Verification items for the finished model (mm, model axes). A direction names the side the tool comes from. Give positions to 0.01 mm unless a question says otherwise; leave off trailing zeros. Loops run counter-clockwise (first coordinate to the right, second up) from the corner with the lowest first, then second, coordinate; pieces in that order, holes last. Notation, with made-up numbers: M 15.5,-24.75 L 32.5,-24.75 A34 cw 32.5,9.25 Z; hole C -32.5,-9 d2. An arc over 180 degrees is marked long. Write each question's results on one line, items separated by ' | '. Start each with the question number.
Autodesk Inventor part; units mm, degrees
ref_plane "YZ Plane" through (0, 0, 0) normal (1, 0, 0) x (0, 1, 0)
ref_plane "XZ Plane" through (0, 0, 0) normal (0, 1, 0) x (-1, 0, 0)
ref_plane "XY Plane" through (0, 0, 0) normal (0, 0, 1) x (1, 0, 0)
sketch "Sketch1" plane through (0, 0, 0) normal (1, 0, 0) x (0, 1, 0)
  line L0 (0, 0) -> (19, 0)
  line L1 (19, 0) -> (19, -9)
  line L2 (19, -9) -> (10.3, -9)
  line L3 (10.3, -9) -> (10.3, -14)
  line L4 (10.3, -14) -> (8.65, -14)
  line L5 (8.65, -14) -> (8.65, -12.5)
  line L6 (8.65, -12.5) -> (1.65, -12.5)
  line L7 (1.65, -12.5) -> (1.65, -14)
  line L8 (1.65, -14) -> (0, -14)
  line L9 (0, -14) -> (0, 0)
  line L10 (0, -5) -> (19, -5)
  point P0 (14.65, -9)
  point P1 (9.5, -5)
  dimension "d0" = 19
  dimension "d1" = 18
  dimension "d2" = 28
  dimension "d3" = 7
  dimension "d4" = 8.7
  dimension "d5" = 10
  dimension "d6" = 25
revolve "Revolution1" add sketch "Sketch1" angle 360 about axis through (0, 0, 0) along (0, 1, 0) contours L10 L1 L2 L3 L4 L5 L6 L7 L8 L9
properties part number "Z Axis Belt Pulley" material "Aluminum 6061"
1. Set-up check for faces 4 (the face through (8.923, 14.589, 1.172)), 5 (the face through (-11.5, 1.65, 5.3)), 6 (the face through (6, 0, 0)): record each of +Z, -Z, +X, -X, +Y, -Y from which the full face is reachable in a straight line by a thin tool's end or side.
2. Section check C-C, the plane y = 16. Record the boundary of the cut face in (x, z).
3. Thickness scan on probe 1 along X at (y, z) = (12.25, 0); probe 2 along X at (y, z) = (2, 0.25). Record the ranges inside material, lowest first.
4. Section check D-D, the plane z = 5.75. Record the boundary of the cut face in (x, y), plus the area to 3 significant figures.
5. Depth check by flat-ended pin: pin 1 Ø4 at (x, y) = (-5, 9) entering from +Z; pin 2 Ø6 at (x, z) = (0, 0) entering from -Y; pin 3 Ø6 at (y, z) = (8, 10.5) entering from +X; pin 4 Ø8 at (y, z) = (10.5, -10.5) entering from -X. Enter the tip coordinate at first touch or a pass-through.
6. Section check B-B, the plane z = 0. Record the boundary of the cut face in (x, y).
7. Release check for a two-part mould opening along Y. For faces 1 (the face through (3, 10.3, -9)), 2 (the face through (-11.5, 8.65, 5.3)), 3 (the face through (4.88, 9.63, 1.08)) record: released by +Y, released by -Y, zero draft, split by the parting line, or undercut.
8. Section check A-A, the plane x = 0. Record the boundary of the cut face in (y, z), plus the area to 3 significant figures.
Filled sheet:
1) face 4: +Y | face 5: none | face 6: +Z, -Z, +X, -X, -Y
2) outline: C 0,0 d18; hole C 0,0 d10
3) probe 1: -9 to -5, 5 to 9 | probe 2: -12.5 to -4.99, 4.99 to 12.5
4) outline: M -12.76,0 L 12.76,0 L 12.76,1.65 L 11.1,1.65 L 11.1,8.65 L 12.76,8.65 L 12.76,10.3 L 6.92,10.3 L 6.92,19 L -6.92,19 L -6.92,10.3 L -12.76,10.3 L -12.76,8.65 L -11.1,8.65 L -11.1,1.65 L -12.76,1.65 Z | area: 360 mm2
5) pin 1: z = 13.67 | pin 2: through | pin 3: x = 11.78 | pin 4: x = -12.4
6) outline: M -14,0 L -5,0 L -5,19 L -9,19 L -9,10.3 L -14,10.3 L -14,8.65 L -12.5,8.65 L -12.5,1.65 L -14,1.65 Z; M 5,0 L 14,0 L 14,1.65 L 12.5,1.65 L 12.5,8.65 L 14,8.65 L 14,10.3 L 9,10.3 L 9,19 L 5,19 Z
7) face 1: released by +Y | face 2: undercut | face 3: zero draft
8) outline: M 0,-14 L 1.65,-14 L 1.65,-12.5 L 8.65,-12.5 L 8.65,-14 L 10.3,-14 L 10.3,-9 L 19,-9 L 19,-5 L 0,-5 Z; M 0,5 L 19,5 L 19,9 L 10.3,9 L 10.3,14 L 8.65,14 L 8.65,12.5 L 1.65,12.5 L 1.65,14 L 0,14 Z | area: 234 mm2
